Read the model definition and answer for the solid it produces. Units are mm, in the model's axes. A direction names the side the tool comes from. Round coordinates to 2 decimals unless told otherwise and drop trailing zeros. Loops run counter-clockwise (first coordinate to the right, second up) from the corner with the lowest first, then second, coordinate; pieces in that order, holes last. Notation, with made-up numbers: M -11,-29.5 L 21,-29.5 A25 cw 21,1.5 Z; hole C 71.25,37.5 d2. An arc over 180 degrees is marked long. Answer as CSV lines item,"result".
Autodesk Fusion 360 part; units mm, degrees
sketch "Sketch1" plane through (0, 0, 0) normal (0, 1, 0) x (1, 0, 0)
  line L0 (0, 0) -> (14, 0)
  line L1 (14, 0) -> (14, 6)
  line L2 (14, 6) -> (0, 6)
  line L3 (0, 6) -> (0, 0)
  dimension "d1" = 14
  dimension "d2" = 6
extrude "Extrude1" add sketch "Sketch1" along normal blind 10
sketch "Sketch2" plane through (0, 10, 0) normal (0, 1, 0) x (-1, 0, 0)
  line L0 (0, -6) -> (0, 0)
  line L1 (0, 0) -> (-14, 0)
  line L2 (-14, 0) -> (-14, -6)
  line L3 (-14, -6) -> (0, -6)
  line L4 (-2, -4) -> (-12, -4)
  line L5 (-12, -4) -> (-12, -2)
  line L6 (-12, -2) -> (-2, -2)
  line L7 (-2, -2) -> (-2, -4)
  dimension "d5" = 2
  dimension "d6" = 2
  dimension "d7" = 2
  dimension "d8" = 2
extrude "Extrude2" add sketch "Sketch2" along normal blind 3 contours L4 L5 L6 L7
1) Find section D-D, the plane x = 13.25. Give the vertices of the cut face in (y, z), then the cut area to 3 significant figures.
Evaluation:
outline,"M 0,-6 L 10,-6 L 10,0 L 0,0 Z"
area,"60.0 mm^2"
2) Find section C-C, the plane y = 12. Give the vertices of the cut face in (x, z).
Evaluation:
outline,"M 2,-4 L 12,-4 L 12,-2 L 2,-2 Z"
3) A tool of negligible diameter and unlimited length cuts with its end or side. For faces 1 (the flat face through (12, 11, -3)), 2 (the flat face through (7, 11, -2)), 3 (the flat face through (2, 11, -3)), 4 (the flat face through (7, 11, -4)), from which of +Z, -Z, +X, -X, +Y, -Y can it reach the whole face along a straight path? Write none if from no direction.
Evaluation:
face 1,"+Z, -Z, +X, +Y"
face 2,"+Z, +X, -X, +Y"
face 3,"+Z, -Z, -X, +Y"
face 4,"-Z, +X, -X, +Y"
4) Each of these flat-tipped pins is pushed along its axis until it touches: P1, Ø1.6, axis at y = 12, z = -3.5, coming from the -X side; P2, Ø2.5, axis at x = 6.5, y = 11.5, coming from the +Z side; P3, Ø0.9, axis at x = 9, y = 12, coming from the -Z side. Where does it stop, or does it pass through?
Evaluation:
P1,"stops at x = 2"
P2,"stops at z = -2"
P3,"stops at z = -4"
5) Find section A-A, the plane x = 4.5. Give the vertices of the cut face in (y, z).
Evaluation:
outline,"M 0,-6 L 10,-6 L 10,-4 L 13,-4 L 13,-2 L 10,-2 L 10,0 L 0,0 Z"
6) Find section B-B, the plane z = -2.35. Give the vertices of the cut face in (x, y).
Evaluation:
outline,"M 0,0 L 14,0 L 14,10 L 12,10 L 12,13 L 2,13 L 2,10 L 0,10 Z"
7) Straight lines are drawn through the part: line 1 (X direction, y = 10.25, z = -2.95); line 2 (Z direction, x = 9.5, y = 10.5); line 3 (Y direction, x = 12.75, z = -0.75). For each, find the intervals that lie inside material, in ascending order.
Evaluation:
line 1,"x = 2 to 12"
line 2,"z = -4 to -2"
line 3,"y = 0 to 10"
